The listing builds one solid part. Answer for the finished solid, in the listing's coordinates (mm). Round coordinates to 2 decimals unless told otherwise and drop trailing zeros. Order: outer loops, then holes, each group sorted by start corner. A loop starts at its lowest first (then second) coordinate and runs counter-clockwise, first axis right, second up. Notation, with made-up numbers: (21.5, 6.5) -> (65.5, 6.5) arc R25 cw to (65.5, 27.5) -> close; hole circle Ø2 at (82, 62.25). An arc over 180 degrees is marked (long way). Answer in a Markdown table with one row per item. Add a question column.
```python
from build123d import *

# Parameters (mm, degrees)
SKETCH1_R           = 10.033
BOSS_EXTRUDE1_DEPTH = 25.019
SKETCH2_R           = 4
CUT_EXTRUDE1_DEPTH  = 10.16
SKETCH3_R           = 4.7625
CUT_EXTRUDE2_DEPTH  = 14.859


with BuildPart() as part:
    # Sketch1 → Boss-Extrude1 (new body)
    with BuildSketch(Plane(origin=(0, 0, 0), x_dir=(1, 0, 0), z_dir=(0, 1, 0))):
        Circle(SKETCH1_R)
    extrude(amount=BOSS_EXTRUDE1_DEPTH)

    # Sketch2 → Cut-Extrude1 (cut)
    with BuildSketch(Plane.XZ):
        Circle(SKETCH2_R)
    extrude(amount=-CUT_EXTRUDE1_DEPTH, mode=Mode.SUBTRACT)

    # Sketch3 → Cut-Extrude2 (cut)
    with BuildSketch(Plane(origin=(0, 25.019, 0), x_dir=(1, 0, 0), z_dir=(0, 1, 0))):
        Circle(SKETCH3_R)
    extrude(amount=-CUT_EXTRUDE2_DEPTH, mode=Mode.SUBTRACT)


solid = part.part
```
Item 1: Find the intervals of material crossed by probe 1 along Z at (x, y) = (0, 7.5); probe 2 along X at (y, z) = (20.25, 0), in increasing order. Write a range as [from, to].
Item 2: The part is cut by section C-C, the plane y = 18. Give the vertices of the cut face in (x, z) (1 decimal), and give its area (3 significant figures).
Item 3: The part is cut by section A-A, the plane x = 0. Give the vertices of the cut face in (y, z).
Item 4: The part is cut by section D-D, the plane x = 8.75. Give the vertices of the cut face in (y, z), and give its area (3 significant figures).
Item 5: The part is cut by section B-B, the plane z = 0. Give the vertices of the cut face in (x, y).
Item 6: For a pull along Z with two mould halves and no side action, classify faces 1 (the face through (4.3, 25.019, -2.4)), 2 (the face through (-2.175, 12.334, 9.794)), 3 (the face through (-3.78, 17.69, 2.9)) as released by +Z, released by -Z, zero draft, split by the parting line, or undercut.
Item 7: Flat-ended cylindrical pins translate along their axes: P1, Ø5, axis at x = 0.5, z = 0, coming from the +Y side; P2, Ø1, axis at x = -3, y = 6.5, coming from the -Z side; P3, Ø8.5, axis at x = 0, z = 0, coming from the +Y side. Find the tip coordinate at first contact, or state that the pin passes through.
Resolved:
| question | item | result |
|---|---|---|
| 1 | probe 1 | [-10.03, -4], [4, 10.03] |
| 1 | probe 2 | [-10.03, -4.76], [4.76, 10.03] |
| 2 | outline | circle Ø20.1 at (0, 0); hole circle Ø9.5 at (0, 0) |
| 2 | area | 245 mm2 |
| 3 | outline | (0, -10.03) -> (25.02, -10.03) -> (25.02, -4.76) -> (10.16, -4.76) -> (10.16, -4) -> (0, -4) -> close; (0, 4) -> (10.16, 4) -> (10.16, 4.76) -> (25.02, 4.76) -> (25.02, 10.03) -> (0, 10.03) -> close |
| 4 | outline | (0, -4.91) -> (25.02, -4.91) -> (25.02, 4.91) -> (0, 4.91) -> close |
| 4 | area | 246 mm2 |
| 5 | outline | (-10.03, 0) -> (-4, 0) -> (-4, 10.16) -> (-4.76, 10.16) -> (-4.76, 25.02) -> (-10.03, 25.02) -> close; (4, 0) -> (10.03, 0) -> (10.03, 25.02) -> (4.76, 25.02) -> (4.76, 10.16) -> (4, 10.16) -> close |
| 6 | face 1 | zero draft |
| 6 | face 2 | split by the parting line |
| 6 | face 3 | undercut |
| 7 | P1 | through |
| 7 | P2 | z = -9.72 |
| 7 | P3 | y = 10.16 |
